Verification items for the finished model (mm, model axes). A direction names the side the tool comes from. Coordinates: 2 decimals unless noted, no trailing zeros. Write each loop counter-clockwise with the first axis right and the second up, starting at its lowest first coordinate (ties: lowest second). Pieces come first, ordered by that corner, then holes.
Autodesk Inventor part; units mm, degrees
ref_plane "YZ Plane" through (0, 0, 0) normal (1, 0, 0) x (0, 1, 0)
ref_plane "XZ Plane" through (0, 0, 0) normal (0, 1, 0) x (-1, 0, 0)
ref_plane "XY Plane" through (0, 0, 0) normal (0, 0, 1) x (1, 0, 0)
sketch "Sketch1" plane through (0, 0, 0) normal (0, 0, 1) x (1, 0, 0)
  arc A0 (18.8233, -2.9299) -> (-18.8233, 2.9299) centre (0, 0) ccw
  arc A1 (-52.0289, -210.4013) -> (-14.3822, -216.2611) centre (-33.2055, -213.3312) ccw
  line L0 (0, 0) -> (-33.2055, -213.3312) construction
  line L1 (18.8233, -2.9299) -> (-14.3822, -216.2611)
  line L2 (-18.8233, 2.9299) -> (-52.0289, -210.4013)
  line L3 (-33.2055, -213.3312) -> (-14.3822, -216.2611) construction
  line L4 (0, 0) -> (18.8233, -2.9299) construction
  arc A2 (23.5292, -3.6624) -> (-23.5292, 3.6624) centre (0, 0) ccw
  arc A3 (-56.7347, -209.6688) -> (-9.6763, -216.9936) centre (-33.2055, -213.3312) ccw
  line L5 (-23.5292, 3.6624) -> (-56.7347, -209.6688)
  line L6 (-9.6763, -216.9936) -> (23.5292, -3.6624)
  dimension "d0" = 215.9
  dimension "d1" = 4.7625
  dimension "d2" = 19.05
extrude "Extrusion1" add sketch "Sketch1" along normal blind 4.7625
fillet "Fillet1" radius 2.3813 8 edges at (-36.8679, -236.8604, 4.7625) (-40.1319, -103.0032, 4.7625) (3.6624, 23.5292, 4.7625) (6.9264, -110.328, 4.7625) (3.6624, 23.5292, 0) (-40.1319, -103.0032, 0) (-36.8679, -236.8604, 0) (6.9264, -110.328, 0)
properties part number "Belt_VerticalConveyor_Outer"
1. Material ranges on L1, parallel to X at y = -34, z = 3.15; L2, parallel to X at y = -117, z = 3.4; L3, parallel to Z at x = 8, y = -94.5, recorded low to high.
2. Tool access check on faces 5 (the flat face through (2.453, -108.102, 2.348)), 6 (the flat face through (-37, -106, 0)). Record the directions out of +Z, -Z, +X, -X, +Y, -Y that give a thin tool (end or side, any length) a straight path to the whole face; none if there is none.
3. Draft check along X on faces 1 (the cylindrical face through (-39.693, -104.601, 0.716)), 2 (the cylindrical face through (-35.721, -232.214, 2.348)), 3 (the flat face through (-35.194, -102.242, 2.348)), 4 (the flat face through (-37, -106, 4.762)). Enter one of: pulls with the +X half, pulls with the -X half, needs draft (parallel to the pull), parting line crosses it, or undercut.
4. Sectioned sample at A-A, the plane z = 1.15. Record the boundary of the cut face in (x, y).
5. Gauge pin test, flat end, axial feed: P1, Ø1.5, axis at x = -26.5, y = -55.5, coming from the -Z side. Record the tip position at first contact, or that the pin passes through.
Outcome:
1. L1: x = -29.26 to -24.57, 13.99 to 18.68
1. L2: x = -42.08 to -37.49, 1.07 to 5.66
1. L3: z = 0.22 to 4.54
2. face 5: +Z, -Z
2. face 6: -Z, +X, -X, +Y, -Y
3. face 1: pulls with the -X half
3. face 2: undercut
3. face 3: undercut
3. face 4: needs draft
4. outline: (-56.4, -209.72) arc R23.47 ccw to (-10.02, -216.94) - (23.19, -3.61) arc R23.47 ccw to (-23.19, 3.61) - close; hole (-52.03, -210.4) arc R19.05 ccw to (-14.38, -216.26) - (18.82, -2.93) arc R19.05 ccw to (-18.82, 2.93) - close
5. P1: passes through
